Autodesk Inventor part; units mm, degrees
ref_plane "YZ Plane" through (0, 0, 0) normal (1, 0, 0) x (0, 1, 0)
ref_plane "XZ Plane" through (0, 0, 0) normal (0, 1, 0) x (-1, 0, 0)
ref_plane "XY Plane" through (0, 0, 0) normal (0, 0, 1) x (1, 0, 0)
sketch "Sketch1" plane through (0, 0, 0) normal (0, 0, 1) x (1, 0, 0)
  line L0 (0, 0) -> (7.25, 0)
  line L1 (0, 0) -> (0, 4)
  line L2 (0, 4) -> (6.5, 4)
  line L3 (9.25, 2) -> (9.25, 4.3765)
  arc A0 (11.75, 9.5) -> (9.25, 4.3765) centre (15.75, 4.3765) ccw
  arc A1 (7.25, 0) -> (9.25, 2) centre (7.25, 2) ccw
  line L4 (3.4828, -0.5) -> (32.44, -0.5) construction
  arc A2 (6.5, 4) -> (7, 4.4933) centre (6.5, 4.5) ccw
  line L5 (11.75, 9.5) -> (15.75, 9.5)
  line L6 (15.75, 9.5) -> (15.75, 6.4102) construction
  line L7 (15.75, 9.5) -> (19.75, 9.5)
  arc A3 (22.25, 4.3765) -> (19.75, 9.5) centre (15.75, 4.3765) ccw
  line L8 (22.25, 4.3765) -> (22.25, 2)
  arc A4 (22.25, 2) -> (24.25, 0) centre (24.25, 2) ccw
  line L9 (24.25, 0) -> (31.5, 0)
  line L10 (31.5, 0) -> (31.5, 4)
  line L11 (31.5, 4) -> (25, 4)
  arc A5 (24.5, 4.4933) -> (25, 4) centre (25, 4.5) ccw
  arc A6 (24.5, 4.4933) -> (7, 4.4933) centre (15.75, 4.3765) ccw
  line L12 (3.25, 4) -> (3.25, 2) construction
  line L13 (28.25, 4) -> (28.25, 2.1903) construction
  point P0 (6.9889, 4)
  dimension "d0" = 4
  dimension "d4" = 2
  dimension "d6" = 6.5
  dimension "d7" = 0.5
  dimension "d9" = 0.5
  dimension "d10" = 4
  dimension "d11" = 6.5
  dimension "d12" = 6.5
  dimension "d13" = 10
  dimension "d14" = 25
extrude "Extrusion1" add sketch "Sketch1" along normal blind 10
chamfer "Chamfer1" distance 2 angle 45 4 edges at (0, 2, 10) (0, 2, 0) (31.5, 2, 10) (31.5, 2, 0)
sketch "Sketch2" plane through (6.5, 4, 10) normal (0, 1, 0) x (1, 0, 0)
  line L0 (-6.5, 8) -> (-6.5, 2)
  line L1 (-6.5, 5) -> (25, 5) construction
  line L2 (25, 8) -> (25, 2)
  circle A0 centre (-2.75, 5) radius 3.75 construction
  circle A1 centre (21.25, 5) radius 3.75 construction
  circle A2 centre (-2.75, 5) radius 1.7
  circle A3 centre (21.25, 5) radius 1.7
  line L3 (-2.75, 8.4641) -> (0.25, 6.7321)
  line L4 (0.25, 6.7321) -> (0.25, 3.2679)
  line L5 (0.25, 3.2679) -> (-2.75, 1.5359)
  line L6 (-2.75, 1.5359) -> (-5.75, 3.2679)
  line L7 (-5.75, 3.2679) -> (-5.75, 6.7321)
  line L8 (-5.75, 6.7321) -> (-2.75, 8.4641)
  line L9 (21.25, 8.4641) -> (24.25, 6.7321)
  line L10 (24.25, 6.7321) -> (24.25, 3.2679)
  line L11 (24.25, 3.2679) -> (21.25, 1.5359)
  line L12 (21.25, 1.5359) -> (18.25, 3.2679)
  line L13 (18.25, 3.2679) -> (18.25, 6.7321)
  line L14 (18.25, 6.7321) -> (21.25, 8.4641)
  point P0 (-6.5, 10)
  dimension "d20" = 24
  dimension "d21" = 3.4
  dimension "d22" = 6
extrude "Extrusion2" cut sketch "Sketch2" along normal blind 10 contours A2 | A3 | L3 L4 L5 L6 L7 L8 | L9 L10 L11 L12 L13 L14
extrude "Extrusion3" cut sketch "Sketch2" against normal through all contours A2 | A3
extrude "Extrusion4" cut sketch "Sketch2" against normal blind 1.5 contours A2 | A3 | L3 L4 L5 L6 L7 L8 | L9 L10 L11 L12 L13 L14
properties part number "motor-clamp"
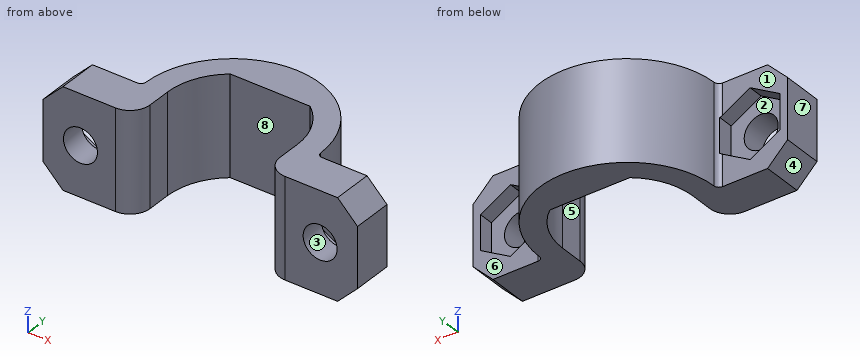
Geometry: final body of the model. Coordinates: model frame, mm. Face numbers are marked on the shaded views. A direction names the side the tool comes from. Coordinates: 2 decimals unless noted, no trailing zeros. Order: outer loops, then holes, each group sorted by start corner. A loop starts at its lowest first (then second) coordinate and runs counter-clockwise, first axis right, second up.
(1) Material intervals for probe 1 along Z at (x, y) = (27.75, 1.55); probe 2 along X at (y, z) = (0.8, 5); probe 3 along X at (y, z) = (1.8, 5), sorted ascending.
(2) Section query B-B (y = 8.25). Return the cut outline in (x, z).
(3) Draft query along X for the marked faces 6, 7 and 8. Return one class per face: pulls with the +X half, pulls with the -X half, needs draft (parallel to the pull), parting line crosses it, or undercut.
(4) Section query D-D (x = 15.75). Return the cut outline in (y, z), plus the area to 3 significant figures.
(5) Access query for the marked faces 1, 2, 3, 4 and 5. Directions: +Z, -Z, +X, -X, +Y, -Y. A direction counts if a zero-diameter tool reaches every point of the face in a straight line with its end or side. Return the directions, or none.
(6) First-contact query: pin 1 (3 mm diameter, centred on x = 15.5, z = 4.5, fed in from +Y); pin 2 (3 mm diameter, centred on x = 3.75, z = 5, fed in from -Y); pin 3 (5 mm diameter, centred on x = 29.5, z = 3, fed in from +Y); pin 4 (3 mm diameter, centred on y = 11, z = 9, fed in from -X). Flat tips, straight axial feed; report the tip coordinate or a pass-through.
(7) Section query A-A (z = 5). State how many separate pieces and enclosed holes the cut face has, plus the area to 3 significant figures.
Solution:
1. probe 1: z = 0 to 3.3, 6.7 to 10
1. probe 2: x = 0 to 2.05, 5.45 to 8.85, 22.65 to 26.05, 29.45 to 31.5
1. probe 3: x = 0 to 2.05, 5.45 to 9.24, 22.26 to 26.05, 29.45 to 31.5
2. outline: (7.9, 0) - (10.53, 0) - (10.53, 10) - (7.9, 10) - close; (20.97, 0) - (23.6, 0) - (23.6, 10) - (20.97, 10) - close
3. face 6: needs draft
3. face 7: pulls with the -X half
3. face 8: undercut
4. outline: (9.5, 0) - (13.13, 0) - (13.13, 10) - (9.5, 10) - close
4. area: 36.3 mm2
5. face 1: +Z, -Z, -X, +Y
5. face 2: +Y
5. face 3: +Y, -Y
5. face 4: -Z, -X, +Y, -Y
5. face 5: +Z, -Z, -Y
6. pin 1: stops at y = 13.13
6. pin 2: passes through
6. pin 3: stops at y = 4
6. pin 4: stops at x = 8.66
7. separate pieces: 3
7. enclosed holes: 0
7. area: 101 mm2
